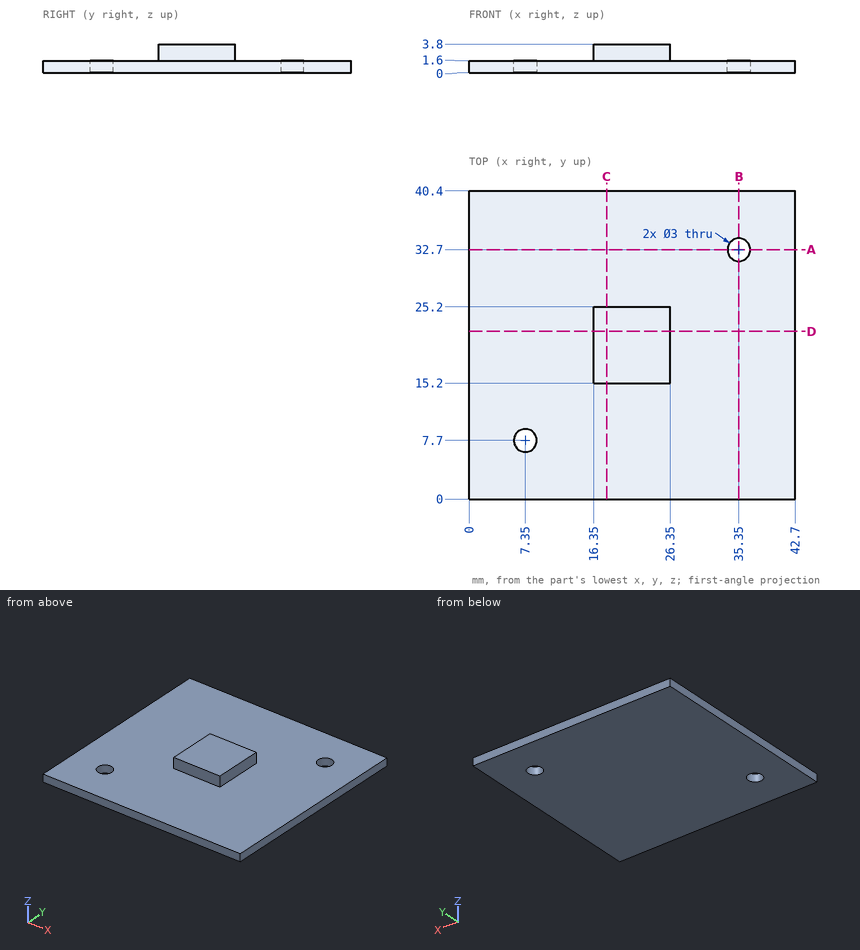
Here's the drawing with two shaded views (mm, measured from the low corner). I have some questions. Give positions to 0.01 mm unless a question says otherwise; leave off trailing zeros. Order: outer loops, then holes, each group sorted by start corner. A loop starts at its lowest first (then second) coordinate and runs counter-clockwise, first axis right, second up. Notation, with made-up numbers: (9.25, 85) - (55.25, 85) arc R13 ccw to (55.25, 105) - close; hole circle Ø9 at (-36, 48.25). An arc over 180 degrees is marked (long way). Use a Markdown table: item, result. Add a question column.
Q1. If we section it at B-B on x = 35.35: Write out the boundary of the cut face in (y, z), plus the area to 3 significant figures.
Q2. If we section it at C-C on x = 18: Write out the boundary of the cut face in (y, z).
Q3. If we section it at D-D on y = 22: Write out the boundary of the cut face in (x, z), plus the area to 3 significant figures.
Q4. Please list where these lines run through material, in increasing order: line 1 along Y through (x, z) = (7.35, 0.9); line 2 along X through (y, z) = (32.7, 0.65); line 3 along Y through (x, z) = (35.35, 0.75).
Q5. If we section it at A-A on y = 32.7: Write out the boundary of the cut face in (x, z), plus the area to 3 significant figures.
Q6. I'm going to push flat-ended pins straight in: pin 1 (2 mm diameter, centred on y = 15, z = 3, fed in from +X); pin 2 (2 mm diameter, centred on x = 19, y = 11.5, fed in from +Z); pin 3 (2.5 mm diameter, centred on x = 7.35, y = 7.7, fed in from -Z); pin 4 (1.8 mm diameter, centred on y = 18, z = 3, fed in from -X). Where does each tip first touch, or does it pass through?
Answers follow:
| question | item | result |
|---|---|---|
| 1 | outline | (0, 0) - (31.2, 0) - (31.2, 1.6) - (0, 1.6) - close; (34.2, 0) - (40.4, 0) - (40.4, 1.6) - (34.2, 1.6) - close |
| 1 | area | 59.8 mm^2 |
| 2 | outline | (0, 0) - (40.4, 0) - (40.4, 1.6) - (25.2, 1.6) - (25.2, 3.8) - (15.2, 3.8) - (15.2, 1.6) - (0, 1.6) - close |
| 3 | outline | (0, 0) - (42.7, 0) - (42.7, 1.6) - (26.35, 1.6) - (26.35, 3.8) - (16.35, 3.8) - (16.35, 1.6) - (0, 1.6) - close |
| 3 | area | 90.3 mm^2 |
| 4 | line 1 | y = 0 to 6.2, 9.2 to 40.4 |
| 4 | line 2 | x = 0 to 33.85, 36.85 to 42.7 |
| 4 | line 3 | y = 0 to 31.2, 34.2 to 40.4 |
| 5 | outline | (0, 0) - (33.85, 0) - (33.85, 1.6) - (0, 1.6) - close; (36.85, 0) - (42.7, 0) - (42.7, 1.6) - (36.85, 1.6) - close |
| 5 | area | 63.5 mm^2 |
| 6 | pin 1 | stops at x = 26.35 |
| 6 | pin 2 | stops at z = 1.6 |
| 6 | pin 3 | passes through |
| 6 | pin 4 | stops at x = 16.35 |
